Could you check a few things on this model? Use its own coordinates, in mm. Face numbers are marked on the shaded views. A direction names the side the tool comes from. Round coordinates to 2 decimals unless told otherwise and drop trailing zeros. Loops run counter-clockwise (first coordinate to the right, second up) from the corner with the lowest first, then second, coordinate; pieces in that order, holes last. Notation, with made-up numbers: (56, 73) -> (114, 73) arc R22 cw to (114, 85) -> close; hole circle Ø11 at (27, 40). An arc over 180 degrees is marked (long way). Write each question's results on one line, items separated by ' | '. Start each with the question number.
1) Imagine slicing it at A-A, the plane z = 206.5. List the corners of the cut face in (x, y) for me, plus the area to 3 significant figures.
2) For P1, Ø10, axis at x = -22, y = -357, coming from the +Z side, with a flat end and sliding along its axis, tell me the tip position at first contact or that it passes through.
3) Which directions (+Z, -Z, +X, -X, +Y, -Y) give clear straight access to the entire face, cutting with the end or side of a thin tool? Please do the marked faces 4 and 5.
4) We'd pull the mould along Z, two halves only. Please class the marked faces 1, 2 and 3: pulls with the +Z half, pulls with the -Z half, needs draft (parallel to the pull), parting line crosses it, or undercut.
5) Imagine slicing it at C-C, the plane y = -74.5. List the corners of the cut face in (x, z) for me, plus the area to 3 significant figures.
6) If I drill on probe 1 along Z at (x, y) = (-59.5, -182); probe 2 along X at (y, z) = (-360, -20); probe 3 along Z at (x, y) = (-120.5, -48.5), over which ranges is the centre line in solid material (lowest first)?
7) Imagine slicing it at B-B, the plane x = 26. List the corners of the cut face in (y, z) for me, plus the area to 3 significant figures.
from build123d import *

# Parameters (mm, degrees)
F0_W        = 330.2
F0_H        = 533.4
F0_W_2      = 279.4
F0_H_2      = 482.6
F1_DEPTH    = 381
F2_R        = 12.7
F3_DEPTH    = 10.16
F4_T1_DEPTH = 635
F4_T3_DEPTH = 584.2


# Not quite as in the source:
# - a fillet or chamfer that OpenCascade refuses, or shapes differently, is made with other operations: its cross-section is extruded or revolved along the edge and cut away or added


with BuildPart() as f1:
    # F0 (on Front) → F1 (new body)
    with BuildSketch(Plane.XZ):
        Rectangle(F0_W, F0_H)
        Rectangle(F0_W_2, F0_H_2, mode=Mode.SUBTRACT)
    extrude(amount=F1_DEPTH)

    # F2 (on face) → F3 (join)
    with BuildSketch(Plane.YZ.offset(165.1)):
        with BuildLine():
            add(Edge.make_bspline(
                [(-378.2229094568, 10.4518691667), (-385.9598838993, 14.4257039209), (-405.6146401633, 14.5371341372), (-437.0263849997, -3.7421973966), (-405.4977582368, -20.7209483443), (-378.1421616626, -20.5633411646), (-363.038665815, -3.6640736551), (-372.1410397823, 7.3281228932), (-378.2229094568, 10.4518691667)],
                knots=[0, 0, 0, 0, 0.1843978335, 0.3570613059, 0.5281889509, 0.7125867844, 0.8550488179, 1, 1, 1, 1], degree=3))
        make_face()
        with Locations((-396.3470816139, -3.5818209283)):
            Circle(F2_R, mode=Mode.SUBTRACT)
    extrude(amount=-F3_DEPTH)

    # F4: fillet of radius 50.8 on 4 edges, made by hand

    # F4_s2 → F4_t1 (cut)
    with BuildSketch(Plane.XZ.offset(-127)):
        with BuildLine():
            ThreePointArc((165.1, 215.9), (150.2210244843, 251.8210244843), (114.3, 266.7))
            Line((114.3, 266.7), (165.1, 266.7))
            Line((165.1, 266.7), (165.1, 215.9))
        make_face()
        with BuildLine():
            ThreePointArc((-165.1, 215.9), (-150.2210244843, 251.8210244843), (-114.3, 266.7))
            Line((-114.3, 266.7), (-165.1, 266.7))
            Line((-165.1, 266.7), (-165.1, 215.9))
        make_face()
    extrude(amount=F4_T1_DEPTH, mode=Mode.SUBTRACT)

    # F4_s4 → F4_t3 (cut)
    with BuildSketch(Plane.YZ.offset(-292.1)):
        with BuildLine():
            ThreePointArc((0, 215.9), (-14.8789755157, 251.8210244843), (-50.8, 266.7))
            Line((-50.8, 266.7), (0, 266.7))
            Line((0, 266.7), (0, 215.9))
        make_face()
        with BuildLine():
            ThreePointArc((-381, 215.9), (-366.1210244843, 251.8210244843), (-330.2, 266.7))
            Line((-330.2, 266.7), (-381, 266.7))
            Line((-381, 266.7), (-381, 215.9))
        make_face()
    extrude(amount=F4_T3_DEPTH, mode=Mode.SUBTRACT)


solid = f1.part
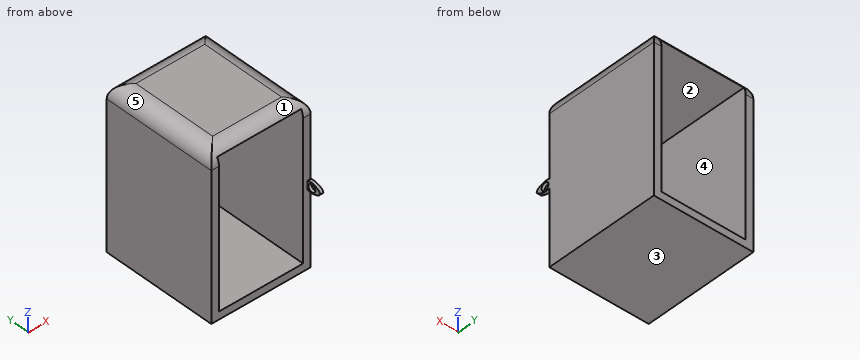
Checked values:
1) outline: (-165.1, -381) -> (-139.7, -381) -> (-139.7, 0) -> (-165.1, 0) -> close; (139.7, -381) -> (165.1, -381) -> (165.1, 0) -> (139.7, 0) -> close | area: 19,400 mm^2
2) P1: z = 261.78
3) face 4: +Y, -Y | face 5: +Z, -X, +Y, -Y
4) face 1: pulls with the +Z half | face 2: undercut | face 3: pulls with the -Z half
5) outline: (-165.1, -266.7) -> (165.1, -266.7) -> (165.1, 215.9) arc R50.8 ccw to (114.3, 266.7) -> (-114.3, 266.7) arc R50.8 ccw to (-165.1, 215.9) -> close; hole (-139.7, -241.3) -> (139.7, -241.3) -> (139.7, 241.3) -> (-139.7, 241.3) -> close | area: 40,200 mm^2
6) probe 1: -266.7 to -241.3, 241.3 to 266.7 | probe 2: -165.1 to -139.7, 139.7 to 165.1 | probe 3: -266.7 to -241.3, 241.3 to 266.32
7) outline: (-381, -266.7) -> (0, -266.7) -> (0, -241.3) -> (-381, -241.3) -> close; (-374.19, 241.3) -> (-6.81, 241.3) arc R50.8 ccw to (-50.8, 266.7) -> (-330.2, 266.7) arc R50.8 ccw to start | area: 18,400 mm^2
